```python
from build123d import *

# Parameters (mm, degrees)
SKETCH1_W               = 16
SKETCH1_H               = 38.42
BOSS_EXTRUDE1_DEPTH     = 2
SKETCH2_W               = 9.5
SKETCH2_H               = 31.92
SKETCH2_W_2             = 6.5
SKETCH2_H_2             = 28.92
EXTRUDE_THIN1_DEPTH     = 2
SKETCH3_R               = 1
CUT_EXTRUDE1_DEPTH      = 5
MIRROR2_COPY_1_SKETCH_R = 1
MIRROR2_COPY_1_DEPTH    = 5
CUT_EXTRUDE_THIN1_START = -1
SKETCH2_3_W             = 9.5
SKETCH2_3_H             = 31.92
SKETCH2_3_W_2           = 6.5
SKETCH2_3_H_2           = 28.92
CUT_EXTRUDE_THIN1_DEPTH = 2
SKETCH5_R               = 0.75
CUT_EXTRUDE2_DEPTH      = 3
CUT_EXTRUDE2_DEPTH_BACK = 3
SKETCH6_R               = 1.25
CUT_EXTRUDE3_DEPTH      = 1


with BuildPart() as part:
    # Sketch1 → Boss-Extrude1 (new body)
    with BuildSketch(Plane(origin=(0, 0, 0), x_dir=(1, 0, 0), z_dir=(0, 1, 0))):
        Rectangle(SKETCH1_W, SKETCH1_H)
    extrude(amount=BOSS_EXTRUDE1_DEPTH)

    # Sketch2 → Extrude-Thin1 (add)
    with BuildSketch(Plane(origin=(0, 2, 0), x_dir=(1, 0, 0), z_dir=(0, 1, 0))):
        Rectangle(SKETCH2_W, SKETCH2_H)
        Rectangle(SKETCH2_W_2, SKETCH2_H_2, mode=Mode.SUBTRACT)
    extrude(amount=EXTRUDE_THIN1_DEPTH)

    # Sketch3 → Cut-Extrude1 (cut, through all)
    with BuildSketch(Plane.XZ):
        with Locations((6, 17.21)):
            Circle(SKETCH3_R)
    cut_extrude1 = extrude(amount=-CUT_EXTRUDE1_DEPTH, mode=Mode.SUBTRACT)

    # Mirror1: Cut-Extrude1 across plane
    add(cut_extrude1.mirror(Plane(origin=(0, 0, 0), x_dir=(1, 0, 0), z_dir=(0, 0, -1))), mode=Mode.SUBTRACT)

    # Mirror2: Cut-Extrude1 across plane
    add(cut_extrude1.mirror(Plane.ZY), mode=Mode.SUBTRACT)

    # Mirror2 copy 1 sketch → Mirror2 copy 1 (cut, through all)
    with BuildSketch(Plane(origin=(0, 0, 0), x_dir=(-1, 0, 0), z_dir=(0, -1, 0))):
        with Locations((6, 17.21)):
            Circle(MIRROR2_COPY_1_SKETCH_R)
    extrude(amount=-MIRROR2_COPY_1_DEPTH, mode=Mode.SUBTRACT)

    # Sketch2<3> → Cut-Extrude-Thin1 (cut)
    with BuildSketch(Plane(origin=(0, 2, 0), x_dir=(1, 0, 0), z_dir=(0, 1, 0)).offset(CUT_EXTRUDE_THIN1_START)):
        Rectangle(SKETCH2_3_W, SKETCH2_3_H)
        Rectangle(SKETCH2_3_W_2, SKETCH2_3_H_2, mode=Mode.SUBTRACT)
    extrude(amount=-CUT_EXTRUDE_THIN1_DEPTH, mode=Mode.SUBTRACT)

    # Sketch5 → Cut-Extrude2 (cut, two sides)
    with BuildSketch(Plane(origin=(0, 2, 0), x_dir=(1, 0, 0), z_dir=(0, 1, 0))) as cut_extrude2_sk:
        Circle(SKETCH5_R)
    extrude(amount=CUT_EXTRUDE2_DEPTH, mode=Mode.SUBTRACT)
    extrude(cut_extrude2_sk.sketch, amount=-CUT_EXTRUDE2_DEPTH_BACK, mode=Mode.SUBTRACT)

    # Sketch6 → Cut-Extrude3 (cut)
    with BuildSketch(Plane.XZ):
        Circle(SKETCH6_R)
    extrude(amount=-CUT_EXTRUDE3_DEPTH, mode=Mode.SUBTRACT)


solid = part.part
```
For this review, take the finished solid that the model builds, in its own axes (mm). A direction names the side the tool comes from. Coordinates: 2 decimals unless noted, no trailing zeros. Write each loop counter-clockwise with the first axis right and the second up, starting at its lowest first coordinate (ties: lowest second). Pieces come first, ordered by that corner, then holes. Notation, with made-up numbers: (-22, -26.75) - (-9, -26.75) arc R10 ccw to (-9, -18.75) - close; hole circle Ø2 at (14.5, -22.75). An arc over 180 degrees is marked (long way). Answer in a Markdown table with one row per item. Add a question column.
Q1. We need section C-C, the plane y = 1.6. State the section outline as (x, z) points.
Q2. Draft analysis for pull direction X (two halves, no side actions). For faces 1 (the flat face through (-0.1, 0.5, -15.96)), 2 (the flat face through (-5, 0, 0)), 3 (the flat face through (-4.75, 3, 0)), state which applies: +X half, -X half, draft (parallel to the pull), parting line (faces both ways), or undercut.
Q3. We need section D-D, the plane x = 0. State the section outline as (y, z) points.
Q4. Tool access review of faces 4 (the cylindrical face through (-5.783, 0.986, -16.234)), 5 (the flat face through (4.75, 0.5, 0.2)), 6 (the flat face through (0, 3, -15.96)), 7 (the flat face through (-3.25, 3, 0)): name each direction out of +Z, -Z, +X, -X, +Y, -Y from which nothing blocks a thin tool from reaching the whole face with its end or side.
Q5. We need section A-A, the plane z = 0. State the section outline as (x, y) points, and give its area (3 significant figures).
Q6. For P1, Ø1.5, axis at x = 6, z = -8, coming from the +Y side; P2, Ø2, axis at x = 0, z = 0, coming from the -Y side; P3, Ø0.6, axis at x = -1, y = 3.5, coming from the -Z side; P4, Ø1, axis at x = 3.5, z = 0.5, coming from the -Y side, all flat-tipped, find the tip position at first contact; note any pin that passes through.
Q7. We need section B-B, the plane x = 6. State the section outline as (y, z) points.
Q8. For probe 1 along Z at (x, y) = (-6, 0.5); probe 2 along Z at (x, y) = (1, 0.75); probe 3 along Z at (x, y) = (2.5, 3.85), list the stretches that pass through material, from the lowest coordinate up.
Answer list:
| question | item | result |
|---|---|---|
| 1 | outline | (-8, -19.21) - (8, -19.21) - (8, 19.21) - (-8, 19.21) - close; hole circle Ø2 at (-6, -17.21); hole circle Ø2 at (-6, 17.21); hole circle Ø1.5 at (0, 0); hole circle Ø2 at (6, -17.21); hole circle Ø2 at (6, 17.21) |
| 2 | face 1 | undercut |
| 2 | face 2 | draft |
| 2 | face 3 | -X half |
| 3 | outline | (0, -19.21) - (2, -19.21) - (2, -15.96) - (4, -15.96) - (4, -14.46) - (2, -14.46) - (2, -0.75) - (1, -0.75) - (1, -1.25) - (0, -1.25) - (0, -14.46) - (1, -14.46) - (1, -15.96) - (0, -15.96) - close; (0, 1.25) - (1, 1.25) - (1, 0.75) - (2, 0.75) - (2, 14.46) - (4, 14.46) - (4, 15.96) - (2, 15.96) - (2, 19.21) - (0, 19.21) - (0, 15.96) - (1, 15.96) - (1, 14.46) - (0, 14.46) - close |
| 4 | face 4 | +Y, -Y |
| 4 | face 5 | -Y |
| 4 | face 6 | -Z, +X, -X, +Y |
| 4 | face 7 | +Y |
| 5 | outline | (-8, 0) - (-4.75, 0) - (-4.75, 1) - (-3.25, 1) - (-3.25, 0) - (-1.25, 0) - (-1.25, 1) - (-0.75, 1) - (-0.75, 2) - (-3.25, 2) - (-3.25, 4) - (-4.75, 4) - (-4.75, 2) - (-8, 2) - close; (0.75, 1) - (1.25, 1) - (1.25, 0) - (3.25, 0) - (3.25, 1) - (4.75, 1) - (4.75, 0) - (8, 0) - (8, 2) - (4.75, 2) - (4.75, 4) - (3.25, 4) - (3.25, 2) - (0.75, 2) - close |
| 5 | area | 31.0 mm2 |
| 6 | P1 | stops at y = 2 |
| 6 | P2 | stops at y = 1 |
| 6 | P3 | stops at z = -15.96 |
| 6 | P4 | stops at y = 0 |
| 7 | outline | (0, -19.21) - (2, -19.21) - (2, -18.21) - (0, -18.21) - close; (0, -16.21) - (2, -16.21) - (2, 16.21) - (0, 16.21) - close; (0, 18.21) - (2, 18.21) - (2, 19.21) - (0, 19.21) - close |
| 8 | probe 1 | z = -19.21 to -18.21, -16.21 to 16.21, 18.21 to 19.21 |
| 8 | probe 2 | z = -19.21 to -15.96, -14.46 to -0.75, 0.75 to 14.46, 15.96 to 19.21 |
| 8 | probe 3 | z = -15.96 to -14.46, 14.46 to 15.96 |
